Here's how the part is built. I have some questions about the finished solid (model axes, mm). A direction names the side the tool comes from. Coordinates: 2 decimals unless noted, no trailing zeros. Write each loop counter-clockwise with the first axis right and the second up, starting at its lowest first coordinate (ties: lowest second). Pieces come first, ordered by that corner, then holes.
Item 1: If I drill on line 1 (X direction, y = 66.5, z = 4.45); line 2 (Z direction, x = -10, y = 2.5); line 3 (Z direction, x = 0, y = 68), over which ranges is the centre line in solid material (lowest first)?
Item 2: If we section it at B-B (z = -10): Please give me the cut outline in (x, y), then the cut area to 4 significant figures.
Item 3: If we section it at C-C (x = 0): Please give me the cut outline in (y, z), then the cut area to 3 significant figures.
Item 4: We'd pull the mould along Z, two halves only. Please class faces 1 (the face through (0, 39, -15)), 2 (the face through (0, 13, 0)), 3 (the face through (0, 39, 15)), 4 (the face through (-0.738, 69.353, 6.795)): +Z half, -Z half, draft (parallel to the pull), parting line (faces both ways), or undercut.
Item 5: If we section it at A-A (x = 10): Please give me the cut outline in (y, z).
Item 6: I'm going to push a flat-ended pin straight in: pin 1 Ø2.5 at (x, z) = (0.5, 4) entering from +Y. Where does the tip first touch, or does it pass through?
Item 7: For faces 5 (the face through (0, 80, 0)), 6 (the face through (0, 59, 4)), 7 (the face through (10, 11, 10)), which set-ups out of +Z, -Z, +X, -X, +Y, -Y let a thin tool reach every point of the face, with its end or its side?
Autodesk Inventor part; units mm, degrees
ref_plane "YZ Plane" through (0, 0, 0) normal (1, 0, 0) x (0, 1, 0)
ref_plane "XZ Plane" through (0, 0, 0) normal (0, 1, 0) x (-1, 0, 0)
ref_plane "XY Plane" through (0, 0, 0) normal (0, 0, 1) x (1, 0, 0)
sketch "Sketch1" plane through (0, 0, 0) normal (0, 1, 0) x (-1, 0, 0)
  line L0 (15, 15) -> (-15, 15)
  line L1 (-15, 15) -> (-15, -15)
  line L2 (-15, -15) -> (15, -15)
  line L3 (15, -15) -> (15, 15)
  line L4 (15, 15) -> (-15, -15) construction
  line L5 (-15, 15) -> (15, -15) construction
  point P0 (0, 0)
  dimension "d0" = 30
  dimension "d1" = 30
extrude "Extrusion1" add sketch "Sketch1" along normal blind 80
sketch "Sketch2" plane through (0, 80, 0) normal (0, 1, 0) x (1, 0, 0)
  line L0 (-15, -15) -> (15, -15) construction
  line L1 (0, -15) -> (0, 3.55) construction
  line L2 (0, 3.55) -> (0, -4.45) construction
  point P0 (0, 0)
  dimension "d4" = 18.55
  dimension "d5" = 8
hole "Hole1" at (0, 80, 4.45) direction (0, -1, 0) diameter 4.917 depth 21
sketch "Sketch3" plane through (0, 0, 0) normal (0, -1, 0) x (1, 0, 0)
  line L0 (-10, -10) -> (10, -10) construction
  line L1 (10, -10) -> (10, 10) construction
  line L2 (10, 10) -> (-10, 10) construction
  line L3 (-10, 10) -> (-10, -10) construction
  line L4 (-10, -10) -> (10, 10) construction
  line L5 (10, -10) -> (-10, 10) construction
  circle A0 centre (10, 10) radius 2.5
  circle A1 centre (-10, -10) radius 2.5
  point P0 (0, 0)
  dimension "d20" = 20
  dimension "d21" = 20
  dimension "d22" = 5
  dimension "d23" = 5
hole "Hole2" at (0, 0, 0) direction (0, 1, 0) diameter 4.917 depth 13
extrude "Extrusion2" cut sketch "Sketch3" against normal blind 11
sketch "Sketch7" plane through (0, 0, 0) normal (0, -1, 0) x (1, 0, 0)
  point P0 (0, 0)
properties part number "TallTower"
Answer list:
1. line 1: x = -15 to -2.46, 2.46 to 15
1. line 2: z = -15 to -12.5, -7.5 to 15
1. line 3: z = -15 to 1.99, 6.91 to 15
2. outline: (-15, 0) - (-12.5, 0) - (-12.5, 11) - (-7.5, 11) - (-7.5, 0) - (15, 0) - (15, 80) - (-15, 80) - close
2. area: 2,345 mm2
3. outline: (0, -15) - (80, -15) - (80, 1.99) - (59, 1.99) - (59, 6.91) - (80, 6.91) - (80, 15) - (0, 15) - (0, 2.46) - (13, 2.46) - (13, -2.46) - (0, -2.46) - close
3. area: 2,230 mm2
4. face 1: -Z half
4. face 2: undercut
4. face 3: +Z half
4. face 4: undercut
5. outline: (0, -15) - (80, -15) - (80, 15) - (0, 15) - (0, 12.5) - (11, 12.5) - (11, 7.5) - (0, 7.5) - close
6. pin 1: stops at y = 59
7. face 5: +Z, -Z, +X, -X, +Y
7. face 6: +Y
7. face 7: -Y
